Model file for the job. Use its own axes, mm. A direction names the side the tool comes from. Coordinates: 2 decimals unless noted, no trailing zeros. Loops run counter-clockwise (first coordinate to the right, second up) from the corner with the lowest first, then second, coordinate; pieces in that order, holes last.
from build123d import *

# Parameters (mm, degrees)
SKETCH1_W           = 30
SKETCH1_H           = 30
BOSS_EXTRUDE1_DEPTH = 1.6
SKETCH2_R           = 0.6
CUT_EXTRUDE1_DEPTH  = 1.6
CIRPATTERN1_COUNT   = 2
CIRPATTERN1_ANGLE   = 90
SKETCH4_R           = 0.6
BOSS_EXTRUDE2_DEPTH = 5


with BuildPart() as part:
    # Sketch1 → Boss-Extrude1 (new body)
    with BuildSketch(Plane(origin=(0, 0, 0), x_dir=(1, 0, 0), z_dir=(0, 1, 0))):
        with Locations((15, 15)):
            Rectangle(SKETCH1_W, SKETCH1_H)
    extrude(amount=BOSS_EXTRUDE1_DEPTH)

    # Sketch2 → Cut-Extrude1 (cut)
    with BuildSketch(Plane(origin=(0, 1.6, 0), x_dir=(1, 0, 0), z_dir=(0, 1, 0))):
        with Locations((19.25, 7)):
            Circle(SKETCH2_R)
        with Locations((10.75, 7)):
            Circle(SKETCH2_R)
        with Locations((19.25, 23)):
            Circle(SKETCH2_R)
        with Locations((10.75, 23)):
            Circle(SKETCH2_R)
    cut_extrude1 = extrude(amount=-CUT_EXTRUDE1_DEPTH, mode=Mode.SUBTRACT)

    # CirPattern1: Cut-Extrude1 ×2 about axis
    cirpattern1_axis = Axis((15, 0, -15), (0, 1, 0))
    for i in range(1, CIRPATTERN1_COUNT):
        add(cut_extrude1.rotate(cirpattern1_axis, i * CIRPATTERN1_ANGLE / (CIRPATTERN1_COUNT - 1)), mode=Mode.SUBTRACT)

    # Sketch4 → Boss-Extrude2 (add)
    with BuildSketch(Plane(origin=(0, 1.6, 0), x_dir=(1, 0, 0), z_dir=(0, 1, 0))):
        with Locations((15, 15)):
            Circle(SKETCH4_R)
    extrude(amount=BOSS_EXTRUDE2_DEPTH)


solid = part.part
Q1. Slice it at C-C (z = -15). List the corners of the cut face in (x, y).
Answers:
outline: (0, 0) - (30, 0) - (30, 1.6) - (15.6, 1.6) - (15.6, 6.6) - (14.4, 6.6) - (14.4, 1.6) - (0, 1.6) - close
Q2. Slice it at D-D (x = 15). List the corners of the cut face in (y, z), and give its area (3 significant figures).
Answers:
outline: (0, -30) - (1.6, -30) - (1.6, -15.6) - (6.6, -15.6) - (6.6, -14.4) - (1.6, -14.4) - (1.6, 0) - (0, 0) - close
area: 54.0 mm2
Q3. Slice it at A-A (z = -10.75). List the corners of the cut face in (x, y).
Answers:
outline: (0, 0) - (6.4, 0) - (6.4, 1.6) - (0, 1.6) - close; (7.6, 0) - (22.4, 0) - (22.4, 1.6) - (7.6, 1.6) - close; (23.6, 0) - (30, 0) - (30, 1.6) - (23.6, 1.6) - close
Q4. Drill centre lines: line 1 (X direction, y = 1.2, z = -23); line 2 (X direction, y = 0.9, z = -19.25); line 3 (Z direction, x = 19.25, y = 1.35). Where is each one in solid material? Low to high.
Answers:
line 1: x = 0 to 10.15, 11.35 to 18.65, 19.85 to 30
line 2: x = 0 to 6.4, 7.6 to 22.4, 23.6 to 30
line 3: z = -30 to -23.6, -22.4 to -7.6, -6.4 to 0
Q5. Which spindle directions (+Z, -Z, +X, -X, +Y, -Y) get a long thin tool onto all of the face, cutting with end or side? Do faces 1 (the cylindrical face through (15.572, 4.065, -15.18)), 2 (the cylindrical face through (7.23, 0.811, -19.804)). Say none if no direction does.
Answers:
face 1: +Y
face 2: +Y, -Y
Q6. Slice it at B-B (x = 7). List the corners of the cut face in (y, z).
Answers:
outline: (0, -30) - (1.6, -30) - (1.6, -19.85) - (0, -19.85) - close; (0, -18.65) - (1.6, -18.65) - (1.6, -11.35) - (0, -11.35) - close; (0, -10.15) - (1.6, -10.15) - (1.6, 0) - (0, 0) - close
Q7. Mould opens along X. For faces 3 (the flat face through (15, 6.6, -15)), 4 (the cylindrical face through (22.405, 0.811, -10.672)), 5 (the flat face through (0, 1, -15)) say: +X half, -X half, draft (parallel to the pull), parting line (faces both ways), or undercut.
Answers:
face 3: draft
face 4: undercut
face 5: -X half
Q8. Flat gauge pins, fed straight in: P1, Ø1.5, axis at x = 9.5, y = 4, coming from the -Z side; P2, Ø9, axis at x = 9.5, z = -15, coming from the +Y side. Where does each tip first touch, or does it go through?
Answers:
P1: passes through
P2: stops at y = 1.6
